from build123d import *

# Parameters (mm, degrees)
SKETCH_W     = 95
SKETCH_H     = 74
PAD_DEPTH    = 0.76
SKETCH001_R  = 3
SKETCH001_W  = 20
SKETCH001_H  = 50
POCKET_DEPTH = 5
FILLET_R     = 3
FILLET001_R  = 1.5


with BuildPart() as part:
    # Sketch → Pad (new body)
    with BuildSketch(Plane.XY):
        Rectangle(SKETCH_W, SKETCH_H)
    extrude(amount=PAD_DEPTH)

    # Sketch001 → Pocket (cut)
    with BuildSketch(Plane.XY.offset(0.76)):
        with Locations((-44, 32.5)):
            Circle(SKETCH001_R)
        with Locations((44, 32.5)):
            Circle(SKETCH001_R)
        with Locations((44, -32.5)):
            Circle(SKETCH001_R)
        with Locations((-44, -32.5)):
            Circle(SKETCH001_R)
        with Locations((54, 0)):
            Rectangle(SKETCH001_W, SKETCH001_H)
        with Locations((-54, 0)):
            Rectangle(SKETCH001_W, SKETCH001_H)
    extrude(amount=-POCKET_DEPTH, mode=Mode.SUBTRACT)

    # Fillet
    fillet_edges = [part.edges().sort_by_distance(p)[0] for p in [
        (-47.5, 37, 0.38),
        (47.5, 37, 0.38),
        (47.5, -37, 0.38),
        (-47.5, -37, 0.38),
    ]]
    fillet(fillet_edges, radius=FILLET_R)

    # Fillet001
    fillet001_edges = [part.edges().sort_by_distance(p)[0] for p in [
        (47.5, -25, 0.38),
        (44, -25, 0.38),
        (44, 25, 0.38),
        (47.5, 25, 0.38),
        (-44, 25, 0.38),
        (-47.5, 25, 0.38),
        (-44, -25, 0.38),
        (-47.5, -25, 0.38),
    ]]
    fillet(fillet001_edges, radius=FILLET001_R)


solid = part.part
Can you work these out from the model? Positions are in its coordinate system, mm. Give positions to 0.01 mm unless a question says otherwise; leave off trailing zeros. Order: outer loops, then holes, each group sorted by start corner. A loop starts at its lowest first (then second) coordinate and runs counter-clockwise, first axis right, second up. Notation, with made-up numbers: M -1,43.5 L 21,43.5 A14 cw 21,62.5 Z; hole C -20,29 d1. An arc over 180 degrees is marked long. Use a Markdown table: item, result. Add a question column.
Item 1: Suppose I cut it at A-A (y = 32.5). List the corners of the cut face in (x, z) for me.
Item 2: Suppose I cut it at C-C (y = 0). List the corners of the cut face in (x, z) for me, then the cut area to 3 significant figures.
Item 3: We'd pull the mould along Y, two halves only. Please class faces 1 (the cylindrical face through (-47, 32.6, 0.4)), 2 (the cylindrical face through (46.6, 36.14, 0.39)), 3 (the flat face through (-1, 1, 0.76)): +Y half, -Y half, draft (parallel to the pull), parting line (faces both ways), or undercut.
Item 4: Suppose I cut it at B-B (z = 0.5). List the corners of the cut face in (x, y) for me, then the cut area to 3 significant figures.
Item 5: If I drill on L1, parallel to Y at x = 43.5, z = 0.55; L2, parallel to X at y = 2.5, z = 0.3, over which ranges is the centre line in solid material (lowest first)? Write a range as [from, to].
Answer sheet:
| question | item | result |
|---|---|---|
| 1 | outline | M -47.5,0 L -47,0 L -47,0.76 L -47.5,0.76 Z; M -41,0 L 41,0 L 41,0.76 L -41,0.76 Z; M 47,0 L 47.5,0 L 47.5,0.76 L 47,0.76 Z |
| 2 | outline | M -44,0 L 44,0 L 44,0.76 L -44,0.76 Z |
| 2 | area | 66.9 mm² |
| 3 | face 1 | undercut |
| 3 | face 2 | +Y half |
| 3 | face 3 | draft |
| 4 | outline | M -47.5,-34 A3 ccw -44.5,-37 L 44.5,-37 A3 ccw 47.5,-34 L 47.5,-26.5 A1.5 ccw 46,-25 L 45.5,-25 A1.5 cw 44,-23.5 L 44,23.5 A1.5 cw 45.5,25 L 46,25 A1.5 ccw 47.5,26.5 L 47.5,34 A3 ccw 44.5,37 L -44.5,37 A3 ccw -47.5,34 L -47.5,26.5 A1.5 ccw -46,25 L -45.5,25 A1.5 cw -44,23.5 L -44,-23.5 A1.5 cw -45.5,-25 L -46,-25 A1.5 ccw -47.5,-26.5 Z; hole C -44,-32.5 d6; hole C -44,32.5 d6; hole C 44,-32.5 d6; hole C 44,32.5 d6 |
| 4 | area | 6,560 mm² |
| 5 | L1 | y = [-37, -35.46], [-29.54, 29.54], [35.46, 37] |
| 5 | L2 | x = [-44, 44] |
